Study the drawing (mm; zero at the part's minimum x, y, z) and answer. A direction names the side the tool comes from. Round coordinates to 2 decimals unless told otherwise and drop trailing zeros. Order: outer loops, then holes, each group sorted by start corner. A loop starts at its lowest first (then second) coordinate and runs counter-clockwise, first axis right, second up. Notation, with made-up numbers: (-24, -1) - (-1, -1) arc R17 cw to (-1, 14) - close; hole circle Ø2 at (9.25, -27). An arc over 180 degrees is marked (long way). Put each result on its own line as item: value. Start each with the question number.
Q1. Which of the six approach directions +Z, -Z, +X, -X, +Y, -Y give full straight-line access (tool end or side, diameter ignored) to the marked faces 5, 6, 7 and 8?
Q2. Section B-B on x = 37 is taken. Give the vertices of the cut face in (y, z), then the cut area to 3 significant figures.
Q3. Section C-C on y = 72 is taken. Give the vertices of the cut face in (x, z), then the cut area to 3 significant figures.
Q4. For a pull along X with two mould halves and no side action, classify the marked faces 1, 2, 3 and 4 as pulls with the +X half, pulls with the -X half, needs draft (parallel to the pull), parting line crosses it, or undercut.
Q5. Section D-D on z = 11 is taken. Give the vertices of the cut face in (x, y), then the cut area to 3 significant figures.
Q6. Each of these flat-tipped pins is pushed along its axis until it touches: pin 1 Ø1.5 at (x, z) = (7.5, 15.5) entering from -Y; pin 2 Ø2 at (x, z) = (15.5, 21.5) entering from -Y; pin 3 Ø3 at (y, z) = (57.5, 23.5) entering from +X; pin 4 Ø6 at (y, z) = (16, 27) entering from +X. Where does it stop, or does it pass through?
Q7. Section A-A on z = 28.5 is taken. Give the vertices of the cut face in (x, y).
Q8. Find the intervals of material crossed by line 1 along Y through (x, z) = (37, 17.5); line 2 along X through (y, z) = (17.5, 2.5); line 3 along Z through (x, y) = (28, 66.5), in increasing order. Write a range as from..to.
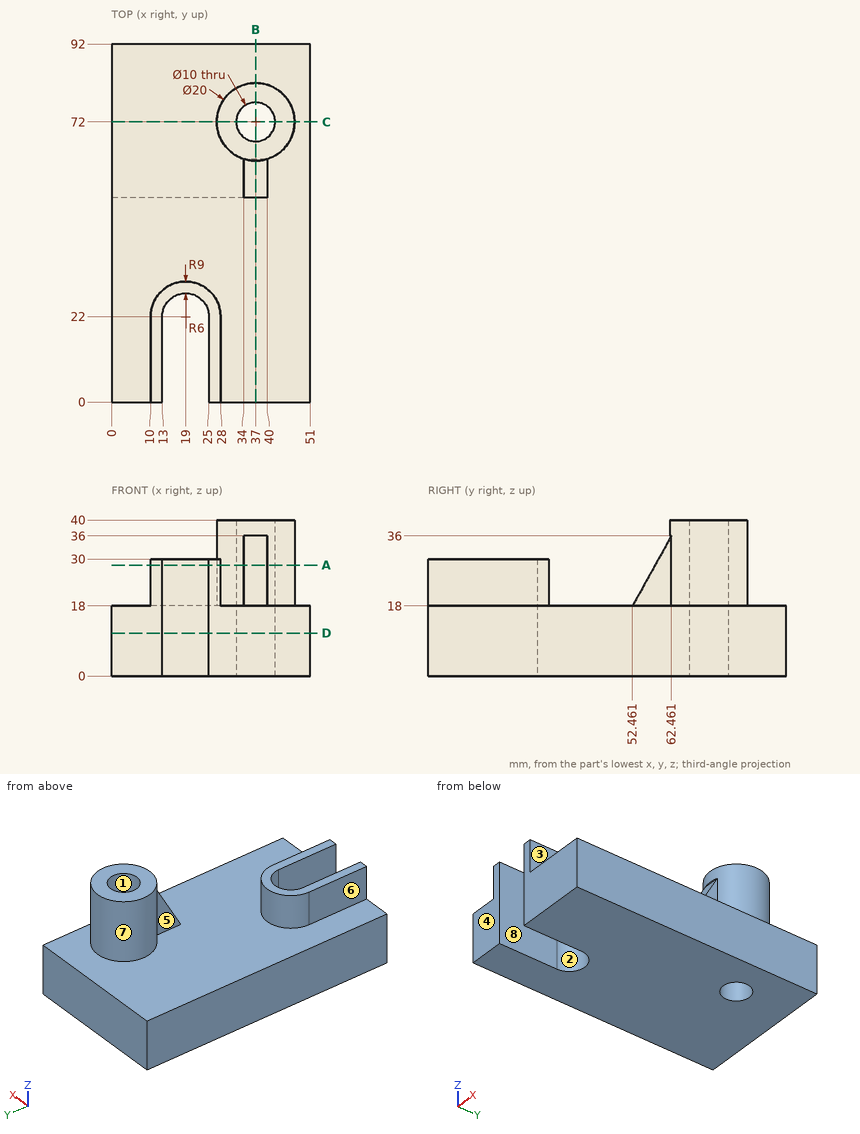
Findings:
1. face 5: +Z, -X, -Y
1. face 6: +Z, -X, +Y, -Y
1. face 7: +Z
1. face 8: +Z, -Z, -Y
2. outline: (0, 0) - (67, 0) - (67, 40) - (62, 40) - (62, 36) - (62.46, 36) - (52.46, 18) - (0, 18) - close; (77, 0) - (92, 0) - (92, 18) - (82, 18) - (82, 40) - (77, 40) - close
2. area: 1,780 mm2
3. outline: (0, 0) - (32, 0) - (32, 40) - (27, 40) - (27, 18) - (0, 18) - close; (42, 0) - (51, 0) - (51, 18) - (47, 18) - (47, 40) - (42, 40) - close
3. area: 958 mm2
4. face 1: undercut
4. face 2: undercut
4. face 3: pulls with the +X half
4. face 4: needs draft
5. outline: (0, 0) - (13, 0) - (13, 22) arc R6 cw to (25, 22) - (25, 0) - (51, 0) - (51, 92) - (0, 92) - close; hole circle Ø10 at (37, 72)
5. area: 4,290 mm2
6. pin 1: y = 0
6. pin 2: y = 25.97
6. pin 3: x = 40
6. pin 4: x = 28
7. outline: (10, 0) - (13, 0) - (13, 22) arc R6 cw to (25, 22) - (25, 0) - (28, 0) - (28, 22) arc R9 ccw to (10, 22) - close; (34, 58.29) - (40, 58.29) - (40, 62.46) arc R10 ccw (long way) to (34, 62.46) - close; hole circle Ø10 at (37, 72)
8. line 1: 0..67, 77..92
8. line 2: 0..13, 25..51
8. line 3: 0..18
